The listing builds one solid part. Answer for the finished solid, in the listing's coordinates (mm). A direction names the side the tool comes from. Coordinates: 2 decimals unless noted, no trailing zeros. Order: outer loops, then holes, each group sorted by start corner. A loop starts at its lowest first (then second) coordinate and runs counter-clockwise, first axis right, second up. Notation, with made-up numbers: (0, 39) - (9, 39) arc R30 cw to (9, 74) - close; hole circle Ø6 at (86.5, -39). An arc over 180 degrees is marked (long way). Use one line per item in the form item = value. Start each with the question number.
Item 1: Each of these flat-tipped pins is pushed along its axis until it touches: pin 1 Ø2.5 at (x, y) = (1, -3) entering from +Z; pin 2 Ø1.5 at (x, y) = (-0.5, -3) entering from -Z; pin 3 Ø5 at (x, z) = (45.3, -0.03) entering from +Y; pin 4 Ø1.5 at (y, z) = (-2, 48) entering from +X. Where does it stop, or does it pass through?
Item 2: The mould has two halves that part along X. Classify faces 3 (the cylindrical face through (43.269, -2.465, -84.554)), 4 (the cylindrical face through (51.59, -2.46, 79.75)), 5 (the flat face through (64.934, -2.535, -37.53)): released by +X, released by -X, zero draft, split by the parting line, or undercut.
Item 3: Section C-C, the plane y = -3.4 is taken. Count the separate pieces of the cut face and the enclosed holes in it, and give its area (3 significant figures).
Item 4: Section A-A, the plane z = 51 is taken. Write down the section's boundary in (x, y).
Item 5: A tool of negligible diameter and unlimited length cuts with its end or side. For faces 1 (the cylindrical face through (27.7, -2.5, 33.2)), 2 (the flat face through (-2.5, -3, 50)), from which of +Z, -Z, +X, -X, +Y, -Y can it reach the whole face along a straight path? Write none if from no direction.
Item 6: Consider line 1 along X through (y, z) = (-1.7, 32); line 2 along Z through (x, y) = (42.5, -3.45); line 3 along Z through (x, y) = (43.5, -1.5). Determine where each line is inside the solid, lowest interval first. Write a range as [from, to].
Item 7: Section B-B, the plane x = 61 is taken. Write down the section's boundary in (y, z), and give its area (3 significant figures).
from build123d import *

# Parameters (mm, degrees)
SKETCH_1_R               = 6
EXTRUDE_1_DEPTH          = 5
CUT_EXTRUDE_1_DEPTH      = 142.435598161
CUT_EXTRUDE_1_DEPTH_BACK = 142.435598161
SKETCH_5_W               = 5
SKETCH_5_H               = 50
F_3_0MM_1_D              = 3
PATTERN_CIRCULAR_1_COUNT = 3
HOLE_WIZARD_M4_1_D       = 3.3


with BuildPart() as part:
    # 草圖1 → 填料-伸長1 (new body)
    with BuildSketch(Plane(origin=(0, 0, 0), x_dir=(1, 0, 0), z_dir=(0, 1, 0))):
        with BuildLine():
            ThreePointArc((-54.140127389, 84.076433121), (-86.602540378, 50), (-99.882390637, 4.848509122))
            ThreePointArc((-99.882390637, 4.848509122), (-94.722486108, -4.890404948), (-83.701905284, -5.024047358))
            ThreePointArc((-83.701905284, -5.024047358), (-32.475952642, -18.75), (-46.201905284, -69.975952642))
            ThreePointArc((-46.201905284, -69.975952642), (-51.596457973, -79.586876805), (-45.742263248, -88.924942243))
            ThreePointArc((-45.742263248, -88.924942243), (0, -100), (45.742263248, -88.924942243))
            ThreePointArc((45.742263248, -88.924942243), (51.596457973, -79.586876805), (46.201905284, -69.975952642))
            ThreePointArc((46.201905284, -69.975952642), (32.475952642, -18.75), (83.701905284, -5.024047358))
            ThreePointArc((83.701905284, -5.024047358), (94.722486108, -4.890404948), (99.882390637, 4.848509122))
            ThreePointArc((99.882390637, 4.848509122), (86.602540378, 50), (54.140127389, 84.076433121))
            ThreePointArc((54.140127389, 84.076433121), (43.126028135, 84.477281753), (37.5, 75))
            ThreePointArc((37.5, 75), (0, 37.5), (-37.5, 75))
            ThreePointArc((-37.5, 75), (-43.126028135, 84.477281753), (-54.140127389, 84.076433121))
        make_face()
        with Locations(Location((0, 0, 0), (0, 0, 270))):
            Circle(SKETCH_1_R, mode=Mode.SUBTRACT)
    extrude(amount=-EXTRUDE_1_DEPTH)

    # 草圖5 → 除料-伸長1 (cut, two sides: drawn at the far end of the back side and taken through both)
    with BuildSketch(Plane(origin=(0, 0, 0), x_dir=(1, 0, 0), z_dir=(0, 1, 0)).offset(-CUT_EXTRUDE_1_DEPTH_BACK)):
        with BuildLine():
            ThreePointArc((18.659757868, -98.243643236), (-14.320442433, -98.969313065), (-45.742263248, -88.924942243))
            ThreePointArc((-45.742263248, -88.924942243), (-51.596457973, -79.586876805), (-46.201905284, -69.975952642))
            ThreePointArc((-46.201905284, -69.975952642), (-35.201155023, -60.328553588), (-28.729686798, -47.205714191))
            ThreePointArc((-28.729686798, -47.205714191), (-19.144613028, -85.825688538), (18.659757868, -98.243643236))
        make_face()
        with BuildLine():
            ThreePointArc((75.751611869, 65.28164596), (92.870160526, 37.082789592), (99.882390637, 4.848509122))
            ThreePointArc((99.882390637, 4.848509122), (94.722486108, -4.890404948), (83.701905284, -5.024047358))
            ThreePointArc((83.701905284, -5.024047358), (69.846637492, -0.320817698), (55.246191092, -1.277781514))
            ThreePointArc((55.246191092, -1.277781514), (83.899533086, 26.333123041), (75.751611869, 65.28164596))
        make_face()
        Polygon((-20.400635095, 14.665063509), (-22.900635095, 10.334936491), (-66.201905284, 35.334936491), (-63.701905284, 39.665063509), align=None)
        with Locations((0, -50)):
            Rectangle(SKETCH_5_W, SKETCH_5_H)
        Polygon((22.900635095, 10.334936491), (20.400635095, 14.665063509), (63.701905284, 39.665063509), (66.201905284, 35.334936491), align=None)
        with BuildLine():
            ThreePointArc((-37.5, 75), (-34.645482469, 60.649371286), (-26.516504294, 48.483495706))
            ThreePointArc((-26.516504294, 48.483495706), (-64.754920057, 59.492565497), (-94.411369737, 32.961997276))
            ThreePointArc((-94.411369737, 32.961997276), (-78.549718093, 61.886523473), (-54.140127389, 84.076433121))
            ThreePointArc((-54.140127389, 84.076433121), (-43.126028135, 84.477281753), (-37.5, 75))
        make_face()
    extrude(amount=CUT_EXTRUDE_1_DEPTH + CUT_EXTRUDE_1_DEPTH_BACK, mode=Mode.SUBTRACT)

    # Ø3.0mm 定位孔1 (through all)
    with Locations(Plane(origin=(0, 0, 0), x_dir=(1, 0, 0), z_dir=(0, 1, 0))):
        with Locations((-36.018712394, 0.206471091), (-22.625047496, -39.249993361), (-77.597265982, 2.931673472)):
            f_3_0mm_1 = Hole(F_3_0MM_1_D / 2)

    # 環狀複製排列1: Ø3.0mm 定位孔1 ×3 about axis
    pattern_circular_1_axis = Axis((0, 0, 0), (0, 1, 0))
    for i in range(1, PATTERN_CIRCULAR_1_COUNT):
        add(f_3_0mm_1.rotate(pattern_circular_1_axis, i * 360 / PATTERN_CIRCULAR_1_COUNT), mode=Mode.SUBTRACT)

    # M4 螺紋孔1 (through all)
    with Locations(Plane(origin=(0, 0, 0), x_dir=(1, 0, 0), z_dir=(0, 1, 0))):
        with Locations((0, 12), (12, 0), (0, -12), (-12, 0)):
            Hole(HOLE_WIZARD_M4_1_D / 2)


solid = part.part
Response:
q1.pin_1 = 98.03
q1.pin_2 = -37.52
q1.pin_3 = 0
q1.pin_4 = 29.18
q2.face_3 = split by the parting line
q2.face_4 = released by +X
q2.face_5 = undercut
q3.separate_pieces = 1
q3.enclosed_holes = 17
q3.area = 15,600 mm2
q4.outline = (-29.56, -5) - (-2.5, -5) - (-2.5, 0) - (-29.56, 0) - close; (2.5, -5) - (29.97, -5) - (29.97, 0) - (2.5, 0) - close
q5.face_1 = +X, +Y, -Y
q5.face_2 = +Y, -Y
q6.line_1 = [-27.86, -2.5], [2.5, 16.51], [19.16, 27.86]
q6.line_2 = [-84.11, -66.68], [-64.79, -27.42], [-21.65, 7.46], [67.54, 90.52]
q6.line_3 = [-84.67, -28], [-22.23, 6.74], [68.26, 90.04]
q7.outline = (-5, -79.24) - (0, -79.24) - (0, -38.11) - (-5, -38.11) - close; (-5, -32.33) - (0, -32.33) - (0, -0.73) - (-5, -0.73) - close
q7.area = 364 mm2
